Geometry check sheet. Reference: drawing and pictorial views, mm from the part's lowest x, y, z. A direction names the side the tool comes from. Coordinates: 2 decimals unless noted, no trailing zeros. Write each loop counter-clockwise with the first axis right and the second up, starting at its lowest first coordinate (ties: lowest second). Pieces come first, ordered by that corner, then holes. Notation, with made-up numbers: (52, 52.5) -> (60, 52.5) arc R29 cw to (60, 86.5) -> close; hole circle Ø6 at (2, 71). An arc over 180 degrees is marked (long way). Use a Markdown table: item, result.
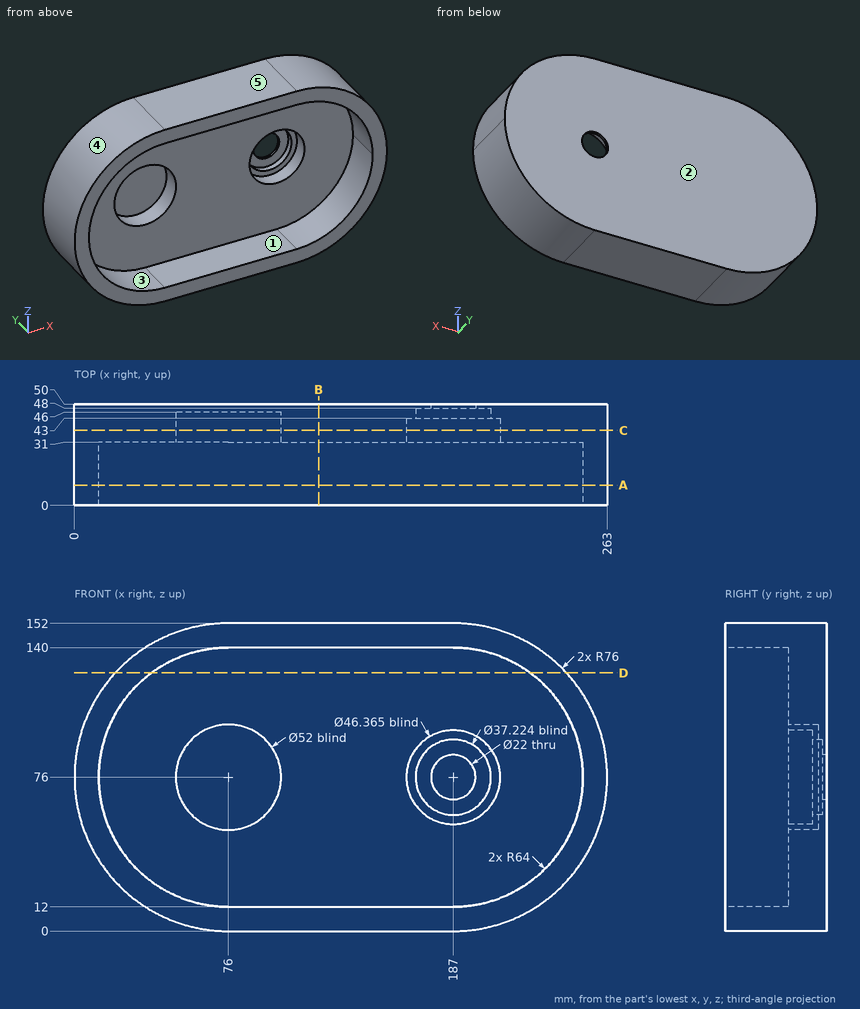
Item 1: Tool access check on the marked faces 1 and 2. Record the directions out of +Z, -Z, +X, -X, +Y, -Y that give a thin tool (end or side, any length) a straight path to the whole face; none if there is none.
Answer block:
| item | result |
|---|---|
| face 1 | -Y |
| face 2 | +Z, -Z, +X, -X, +Y |
Item 2: Thickness scan on L1, parallel to Z at x = 118.5, y = 16; L2, parallel to Z at x = 76, y = 40.5; L3, parallel to Y at x = 142.5, z = 21.5. Record the ranges inside material, lowest first. Write a range as [from, to].
Answer block:
| item | result |
|---|---|
| L1 | z = [0, 12], [140, 152] |
| L2 | z = [0, 50], [102, 152] |
| L3 | y = [31, 50] |
Item 3: Section check A-A on y = 10. Record the boundary of the cut face in (x, z).
Answer block:
| item | result |
|---|---|
| outline | (76, 0) -> (187, 0) arc R76 ccw to (187, 152) -> (76, 152) arc R76 ccw to start; hole (76, 12) -> (187, 12) arc R64 ccw to (187, 140) -> (76, 140) arc R64 ccw to start |
Item 4: Section check C-C on y = 37. Record the boundary of the cut face in (x, z) (1 decimal), then the cut area to 3 significant figures.
Answer block:
| item | result |
|---|---|
| outline | (76, 0) -> (187, 0) arc R76 ccw to (187, 152) -> (76, 152) arc R76 ccw to start; hole circle Ø52 at (76, 76); hole circle Ø46.4 at (187, 76) |
| area | 31,200 mm^2 |
Item 5: Section check D-D on z = 127.5. Record the boundary of the cut face in (x, y).
Answer block:
| item | result |
|---|---|
| outline | (20.11, 0) -> (38, 0) -> (38, 31) -> (225, 31) -> (225, 0) -> (242.89, 0) -> (242.89, 50) -> (20.11, 50) -> close |
Item 6: Mould release check, pull along Z, two halves, no side actions. Record for the marked faces 3, 4 and 5: +Z half, -Z half, draft (parallel to the pull), parting line (faces both ways), or undercut.
Answer block:
| item | result |
|---|---|
| face 3 | undercut |
| face 4 | parting line |
| face 5 | +Z half |
Item 7: Section check B-B on x = 120.5. Record the boundary of the cut face in (y, z), then the cut area to 3 significant figures.
Answer block:
| item | result |
|---|---|
| outline | (0, 0) -> (50, 0) -> (50, 152) -> (0, 152) -> (0, 140) -> (31, 140) -> (31, 12) -> (0, 12) -> close |
| area | 3,630 mm^2 |
Item 8: Depth check by flat-ended pin: P1, Ø8, axis at y = 31.5, z = 130.5, coming from the -X side (1 decimal); P2, Ø6, axis at y = 30, z = 72, coming from the -X side; P3, Ø2, axis at x = 210, z = 107, coming from the -Y side. Enter the tip coordinate at first touch or a pass-through.
Answer block:
| item | result |
|---|---|
| P1 | stops at x = 19.2 |
| P2 | stops at x = 0.01 |
| P3 | stops at y = 31 |
